Drawing for the job (mm, zero at the part's lowest x, y, z). A direction names the side the tool comes from. Round coordinates to 2 decimals unless told otherwise and drop trailing zeros. Write each loop counter-clockwise with the first axis right and the second up, starting at its lowest first coordinate (ties: lowest second). Pieces come first, ordered by that corner, then holes.
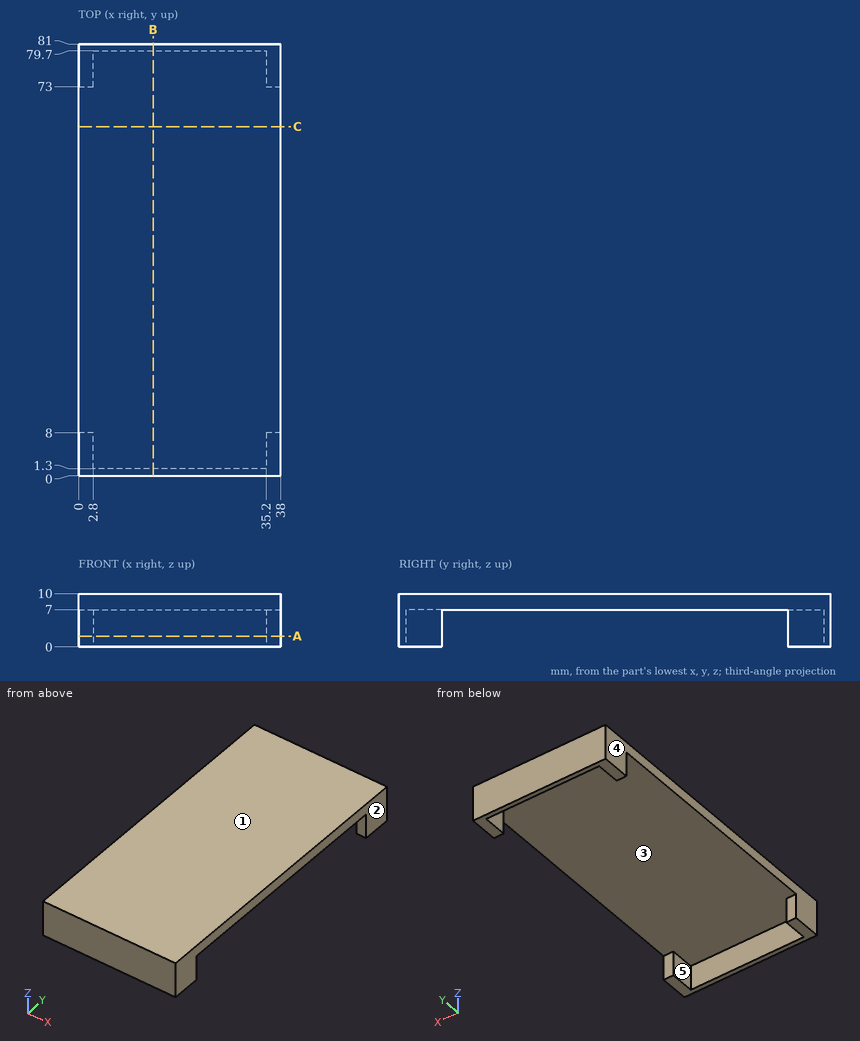
Q1. Two-plate mould, pull along X, no slides. Class the marked faces 1, 2 and 3: released by +X, released by -X, zero draft, split by the parting line, or undercut.
Q2. Saw through at B-B, the plane x = 14. Write the cut outline in (y, z).
Q3. Saw through at C-C, the plane y = 65.5. Write the cut outline in (x, z), and give its area (3 significant figures).
Q4. Wall check: line 1 (Y direction, x = 34.5, z = 4.75); line 2 (Z direction, x = 33, y = 50.5); line 3 (Y direction, x = 35.5, z = 5). Give the ranges that are in metal, low to high.
Q5. Tool access for the marked faces 4 and 5: list every direction of +Z, -Z, +X, -X, +Y, -Y with a clear straight run to the whole face (end or side of a thin tool).
Q6. Saw through at A-A, the plane z = 2. Write the cut outline in (x, y).
Q7. Drop a flat-ended pin along its axis: P1, Ø3, axis at x = 15, y = 44.5, coming from the -Z side. Give the stop position or say it passes through.
Computed:
1. face 1: zero draft
1. face 2: released by +X
1. face 3: undercut
2. outline: (0, 0) - (1.3, 0) - (1.3, 7) - (79.7, 7) - (79.7, 0) - (81, 0) - (81, 10) - (0, 10) - close
3. outline: (0, 7) - (38, 7) - (38, 10) - (0, 10) - close
3. area: 114 mm2
4. line 1: y = 0 to 1.3, 79.7 to 81
4. line 2: z = 7 to 10
4. line 3: y = 0 to 8, 73 to 81
5. face 4: +Z, -Z, -X, +Y, -Y
5. face 5: -Z
6. outline: (0, 0) - (38, 0) - (38, 8) - (35.2, 8) - (35.2, 1.3) - (2.8, 1.3) - (2.8, 8) - (0, 8) - close; (0, 73) - (2.8, 73) - (2.8, 79.7) - (35.2, 79.7) - (35.2, 73) - (38, 73) - (38, 81) - (0, 81) - close
7. P1: stops at z = 7
